Source: CAD feature listing. Evaluate the final solid. Frame: model axes, mm. A direction names the side the tool comes from. Coordinates: 2 decimals unless noted, no trailing zeros. Write each loop counter-clockwise with the first axis right and the second up, starting at its lowest first coordinate (ties: lowest second). Pieces come first, ordered by that corner, then holes. Notation, with made-up numbers: M 29.25,-16.5 L 63.25,-16.5 A13 ccw 63.25,2.5 Z; hole C 69.25,59 d8. An arc over 180 degrees is marked long. Write item = value, one per line. Start each with the question number.
1. Section query C-C (x = 10.25). Output: boundary loops of the cut face in (y, z).
2. Line query: line 1 along X through (y, z) = (4.75, -3.95); line 2 along Z through (x, y) = (7.75, 2.75); line 3 along X through (y, z) = (2.5, -2.75). Output: solid intervals per line, ascending.
3. Access query for faces 1 (the face through (3.8, 6, -2)), 2 (the face through (2, 5, -4)), 3 (the face through (11.7, 6, -6)). Directions: +Z, -Z, +X, -X, +Y, -Y. A direction counts if a zero-diameter tool reaches every point of the face in a straight line with its end or side. Return the directions, or none.
4. Pin query (flat end, axial travel): pin 1 Ø2 at (y, z) = (3, -7) entering from -X; pin 2 Ø1.6 at (y, z) = (6, -6.5) entering from +X; pin 3 Ø0.8 at (y, z) = (6, -1) entering from -X; pin 4 Ø3.5 at (x, z) = (7.75, -3.95) entering from +Y. Return the tip coordinate at first contact, or that it passes through.
5. Section query D-D (z = -6.75). Output: boundary loops of the cut face in (x, y), then the cut area to 3 significant figures.
6. Section query A-A (z = -2.75). Output: boundary loops of the cut face in (x, y).
7. Pull-direction query (Z, two-part tool) for faces 4 (the face through (0, 4.5, -2.7)), 5 (the face through (9.78, 3.2, -6.16)), 6 (the face through (1, 4, -7.4)); classes: pulls with the +Z half, pulls with the -Z half, needs draft (parallel to the pull), parting line crosses it, or undercut.
8. Section query B-B (y = 3.5). Output: boundary loops of the cut face in (x, z).
```python
from build123d import *

# Parameters (mm, degrees)
SKETCH_1_W          = 15.5
SKETCH_1_H          = 7.9
EXTRUDE_1_DEPTH     = 5
EXTRUDE_START       = 5
EXTRUDE_2_DEPTH     = 1.5
CUT_EXTRUDE_2_DEPTH = 19.571752744
CUT_EXTRUDE_3_REACH = 20.572
SKETCH_2_5_R        = 3
CUT_EXTRUDE_4_DEPTH = 19.571752744


with BuildPart() as part:
    # 草图1 → 凸台-拉伸1 (new body)
    with BuildSketch(Plane(origin=(0, 0, 0), x_dir=(1, 0, 0), z_dir=(0, 1, 0))):
        with Locations((7.75, 3.95)):
            Rectangle(SKETCH_1_W, SKETCH_1_H)
    extrude(amount=EXTRUDE_1_DEPTH)

    # 草图2 → 凸台-拉伸2 (add)
    with BuildSketch(Plane(origin=(0, 0, 0), x_dir=(1, 0, 0), z_dir=(0, 1, 0)).offset(EXTRUDE_START)):
        with BuildLine():
            Line((3.8, 3.95), (3.8, 0))
            Line((3.8, 0), (7.75, 0))
            ThreePointArc((7.75, 0), (10.543071786, 1.156928214), (11.7, 3.95))
            Line((11.7, 3.95), (11.7, 7.9))
            Line((11.7, 7.9), (7.75, 7.9))
            ThreePointArc((7.75, 7.9), (4.956928214, 6.743071786), (3.8, 3.95))
        make_face()
    extrude(amount=EXTRUDE_2_DEPTH)

    # 草图3 → 切除-拉伸2 (cut, through all)
    with BuildSketch(Plane.XY):
        Polygon((0, 4.1), (4.1, 0), (0, 0), align=None)
        Polygon((11.4, 0), (15.5, 4.1), (15.5, 0), align=None)
    extrude(amount=-CUT_EXTRUDE_2_DEPTH, mode=Mode.SUBTRACT)

    # 草图4 → 切除-拉伸3 (cut, up to next)
    with BuildSketch(Plane(origin=(0, 0, 0), x_dir=(1, 0, 0), z_dir=(0, 1, 0)), mode=Mode.PRIVATE) as cut_extrude_3_sk1:
        with BuildLine():
            Line((2.5, 7.9), (0, 7.9))
            Line((0, 7.9), (0, 5.4))
            ThreePointArc((0, 5.4), (0.732233047, 7.167766953), (2.5, 7.9))
        make_face()
    cut_extrude_3_tool1 = extrude(cut_extrude_3_sk1.sketch, amount=CUT_EXTRUDE_3_REACH, mode=Mode.PRIVATE) & part.part
    # 草图4 → 切除-拉伸3 (cut, up to next)
    with BuildSketch(Plane(origin=(0, 0, 0), x_dir=(1, 0, 0), z_dir=(0, 1, 0)), mode=Mode.PRIVATE) as cut_extrude_3_sk2:
        with BuildLine():
            Line((13, 0), (15.5, 0))
            Line((15.5, 0), (15.5, 2.5))
            ThreePointArc((15.5, 2.5), (14.767766953, 0.732233047), (13, 0))
        make_face()
    cut_extrude_3_tool2 = extrude(cut_extrude_3_sk2.sketch, amount=CUT_EXTRUDE_3_REACH, mode=Mode.PRIVATE) & part.part
    add(cut_extrude_3_tool1.solids().sort_by_distance((0.55842, 0, -7.34158))[0], mode=Mode.SUBTRACT)
    add(cut_extrude_3_tool2.solids().sort_by_distance((14.94158, 0, -0.55842))[0], mode=Mode.SUBTRACT)

    # 草图2<5> → 切除-拉伸4 (cut, through all)
    with BuildSketch(Plane(origin=(0, 0, 0), x_dir=(1, 0, 0), z_dir=(0, 1, 0))):
        with Locations(Location((7.75, 3.95, 0), (0, 0, 270))):
            Circle(SKETCH_2_5_R)
    extrude(amount=CUT_EXTRUDE_4_DEPTH, mode=Mode.SUBTRACT)


solid = part.part
```
Results are:
q1.outline = M 0,-7.9 L 6.5,-7.9 L 6.5,-5.61 L 0,-5.61 Z; M 0,-2.29 L 6.5,-2.29 L 6.5,-0.89 L 5,-0.89 L 5,0 L 0,0 Z
q2.line_1 = 0 to 4.75, 10.75 to 15.5
q2.line_2 = -7.9 to -6.95, -0.95 to 0
q2.line_3 = 1.6 to 5, 10.5 to 13.9
q3.face_1 = +Z, -Z, -X, +Y
q3.face_2 = -Z, -X, +Y
q3.face_3 = +Z, -Z, +X, +Y
q4.pin_1 = 0.25
q4.pin_2 = 11.7
q4.pin_3 = 3.8
q4.pin_4 = through
q5.outline = M 0.4,3.7 L 4.1,0 L 6.67,0 L 6.67,6.5 L 4.96,6.5 L 4.96,5 L 0.4,5 Z; M 8.83,0 L 11.4,0 L 15.5,4.1 L 15.5,5 L 11.7,5 L 11.7,6.5 L 8.83,6.5 Z
q5.area = 56.4 mm^2
q6.outline = M 0,4.1 L 4.1,0 L 5,0 L 5,6.5 L 3.8,6.5 L 3.8,5 L 0,5 Z; M 10.5,0 L 11.4,0 L 15.5,4.1 L 15.5,5 L 11.51,5 L 11.51,6.5 L 10.5,6.5 Z
q7.face_4 = needs draft
q7.face_5 = undercut
q7.face_6 = pulls with the -Z half
q8.outline = M 0.6,-7.02 A2.5 ccw 2.5,-7.9 L 14.9,-7.9 L 14.9,-0.88 A2.5 ccw 13,0 L 0.6,0 Z; hole C 7.75,-3.95 d6
